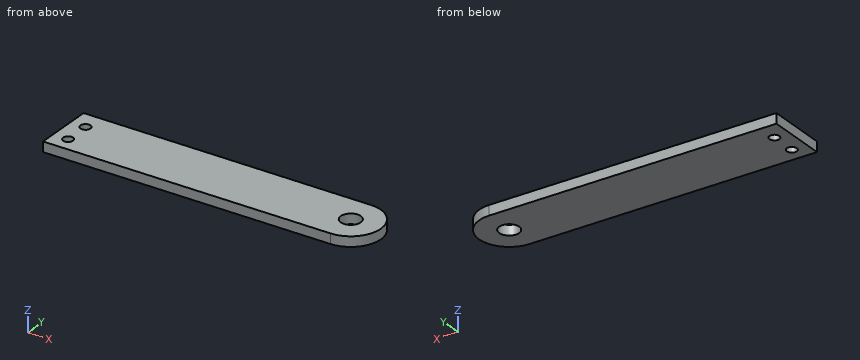
from build123d import *

# Parameters (mm, degrees)
F0_R     = 3.175
F0_R_2   = 6.35
F1_DEPTH = 6.35


with BuildPart() as f1:
    # F0 (on Top) → F1 (new body)
    with BuildSketch(Plane.XY):
        with BuildLine():
            Line((-101.490255, -19.05), (81.072245, -19.05))
            ThreePointArc((81.072245, -19.05), (100.122245, 0), (81.072245, 19.05))
            Line((81.072245, 19.05), (-101.490255, 19.05))
            Line((-101.490255, 19.05), (-101.490255, -19.05))
        make_face()
        with Locations((-91.965255, -9.525)):
            Circle(F0_R, mode=Mode.SUBTRACT)
        with Locations((-91.965255, 6.8072)):
            Circle(F0_R, mode=Mode.SUBTRACT)
        with Locations((81.072245, 0)):
            Circle(F0_R_2, mode=Mode.SUBTRACT)
    extrude(amount=F1_DEPTH)


solid = f1.part
Design review of the part built by this model. Coordinates are the model's own, in mm. Give positions to 0.01 mm unless a question says otherwise; leave off trailing zeros. Loops run counter-clockwise (first coordinate to the right, second up) from the corner with the lowest first, then second, coordinate; pieces in that order, holes last. Notation, with made-up numbers: (-27.5, 28) - (28.5, 28) arc R23 ccw to (28.5, 47) - close; hole circle Ø10 at (79.5, 30.25). An arc over 180 degrees is marked (long way). Use CSV: the item, a comma, the result in double quotes. Start each with the question number.
1. Add section C-C (y = 13.5). State the section outline as (x, z) points, plus the area to 3 significant figures.
2. Add section B-B (z = 5.25). State the section outline as (x, y) points (3 decimals).
3. Insertion check: P1, Ø10, axis at x = -91.97, y = -9.52, coming from the +Z side; P2, Ø3, axis at y = 13, z = 2.5, coming from the +X side. Each pin has a flat end and moves straight along its axis. Give the tip position at first contact, or say it passes through.
4. Wall thickness on L1, parallel to X at y = -0.5, z = 2.25; L2, parallel to X at y = 9, z = 2; L3, parallel to X at y = 5, z = 2.5: over which ranges is each line inside the solid? List them lowest first.
5. Add section A-A (y = 0). State the section outline as (x, z) points.
Results found:
1,outline,"(-101.49, 0) - (94.51, 0) - (94.51, 6.35) - (-101.49, 6.35) - close"
1,area,"1,240 mm²"
2,outline,"(-101.49, -19.05) - (81.072, -19.05) arc R19.05 ccw to (81.072, 19.05) - (-101.49, 19.05) - close; hole circle Ø6.35 at (-91.965, -9.525); hole circle Ø6.35 at (-91.965, 6.807); hole circle Ø12.7 at (81.072, 0)"
3,P1,"stops at z = 6.35"
3,P2,"stops at x = 96.26"
4,L1,"x = -101.49 to 74.74, 87.4 to 100.12"
4,L2,"x = -101.49 to -94.26, -89.67 to 97.86"
4,L3,"x = -101.49 to -94.58, -89.35 to 77.16, 84.99 to 99.45"
5,outline,"(-101.49, 0) - (74.72, 0) - (74.72, 6.35) - (-101.49, 6.35) - close; (87.42, 0) - (100.12, 0) - (100.12, 6.35) - (87.42, 6.35) - close"
